Can you work these out from the model? Positions are in its coordinate system, mm. Round coordinates to 2 decimals unless told otherwise and drop trailing zeros. Write each loop counter-clockwise with the first axis right and the second up, starting at its lowest first coordinate (ties: lowest second). Pieces come first, ordered by that corner, then holes. Notation, with made-up numbers: M -14,55 L 3,55 A19 ccw 3,63 Z; hole C -24,27.5 d1. An arc over 180 degrees is marked long. Answer as a JSON object with one key per item and string values. Group by question number.
1) I'm going to push flat-ended pins straight in: pin 1 Ø3.5 at (x, y) = (8, 8) entering from +Z; pin 2 Ø9.5 at (x, y) = (27.5, 8) entering from +Z. Where does each tip first touch, or does it pass through?
2) Suppose I cut it at B-B, the plane y = 8. Write out the boundary of the cut face in (x, z).
3) Suppose I cut it at C-C, the plane y = 35. Write out the boundary of the cut face in (x, z), and give its area (3 significant figures).
4) Suppose I cut it at A-A, the plane x = 8. Write out the boundary of the cut face in (y, z), and give its area (3 significant figures).
5) Please list where these lines run through material, in increasing order: L1, parallel to X at y = 8, z = -3.5; L2, parallel to Y at x = 27.5, z = 2.75; L3, parallel to Y at x = 8, z = -3. Write a range as [from, to].
6) Suppose I cut it at D-D, the plane x = 27.5. Write out the boundary of the cut face in (y, z).
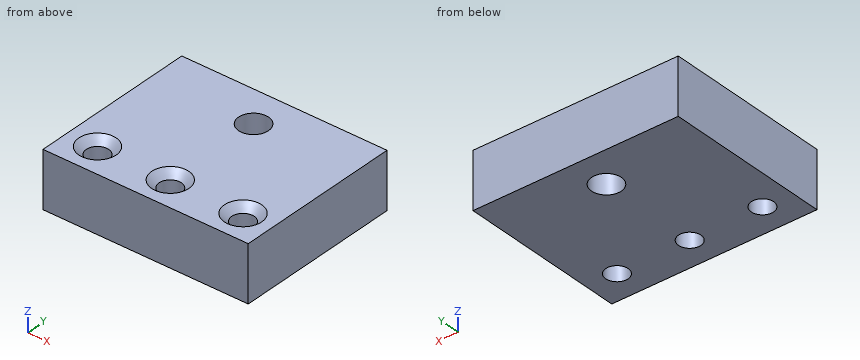
from build123d import *

# Parameters (mm, degrees)
SKETCH1_W                       = 55
SKETCH1_H                       = 45
BOSS_EXTRUDE1_DEPTH             = 7.5
F_6_0MM_DOWEL_HOLE1_D           = 6
F_6_0MM_DOWEL_HOLE1_CSINK_D     = 10
F_6_0MM_DOWEL_HOLE1_CSINK_ANGLE = 90
F_8_0MM_DOWEL_HOLE1_D           = 8


with BuildPart() as part:
    # Sketch1 → Boss-Extrude1 (new body, symmetric)
    with BuildSketch(Plane.XY):
        with Locations((27.5, 22.5)):
            Rectangle(SKETCH1_W, SKETCH1_H)
    extrude(amount=BOSS_EXTRUDE1_DEPTH, both=True)

    # Ø6.0mm Dowel Hole1 (through all)
    with Locations(Plane(origin=(8, 8, 7.5), x_dir=(1, 0, 0), z_dir=(0, 0, 1))):
        with Locations((0, 0), (19.5, 0), (39, 0)):
            CounterSinkHole(F_6_0MM_DOWEL_HOLE1_D / 2, F_6_0MM_DOWEL_HOLE1_CSINK_D / 2, counter_sink_angle=F_6_0MM_DOWEL_HOLE1_CSINK_ANGLE)

    # Ø8.0mm Dowel Hole1 (through all)
    with Locations(Plane(origin=(27.5, 35, 7.5), x_dir=(1, 0, 0), z_dir=(0, 0, 1))):
        with Locations((0, 0)):
            Hole(F_8_0MM_DOWEL_HOLE1_D / 2)


solid = part.part
Results:
{
 "1": {"pin 1": "through", "pin 2": "z = 7.25"},
 "2": {"outline": "M 0,-7.5 L 5,-7.5 L 5,5.5 L 3,7.5 L 0,7.5 Z; M 11,-7.5 L 24.5,-7.5 L 24.5,5.5 L 22.5,7.5 L 13,7.5 L 11,5.5 Z; M 30.5,-7.5 L 44,-7.5 L 44,5.5 L 42,7.5 L 32.5,7.5 L 30.5,5.5 Z; M 50,-7.5 L 55,-7.5 L 55,7.5 L 52,7.5 L 50,5.5 Z"},
 "3": {"outline": "M 0,-7.5 L 23.5,-7.5 L 23.5,7.5 L 0,7.5 Z; M 31.5,-7.5 L 55,-7.5 L 55,7.5 L 31.5,7.5 Z", "area": "705 mm^2"},
 "4": {"outline": "M 0,-7.5 L 5,-7.5 L 5,5.5 L 3,7.5 L 0,7.5 Z; M 11,-7.5 L 45,-7.5 L 45,7.5 L 13,7.5 L 11,5.5 Z", "area": "581 mm^2"},
 "5": {"L1": "[0, 5], [11, 24.5], [30.5, 44], [50, 55]", "L2": "[0, 5], [11, 31], [39, 45]", "L3": "[0, 5], [11, 45]"},
 "6": {"outline": "M 0,-7.5 L 5,-7.5 L 5,5.5 L 3,7.5 L 0,7.5 Z; M 11,-7.5 L 31,-7.5 L 31,7.5 L 13,7.5 L 11,5.5 Z; M 39,-7.5 L 45,-7.5 L 45,7.5 L 39,7.5 Z"}
}
